CAD build for the part. Positions are in the model's coordinates, mm. A direction names the side the tool comes from. Round coordinates to 2 decimals unless told otherwise and drop trailing zeros. Order: outer loops, then holes, each group sorted by start corner. A loop starts at its lowest first (then second) coordinate and runs counter-clockwise, first axis right, second up.
Autodesk Inventor part; units mm, degrees
ref_plane "YZ Plane" through (0, 0, 0) normal (1, 0, 0) x (0, 1, 0)
ref_plane "XZ Plane" through (0, 0, 0) normal (0, 1, 0) x (-1, 0, 0)
ref_plane "XY Plane" through (0, 0, 0) normal (0, 0, 1) x (1, 0, 0)
sketch "Sketch6" plane through (0, 0, 0) normal (1, 0, 0) x (0, 1, 0)
  line L0 (0, 0) -> (12.5, 0)
  line L1 (0, 0) -> (0, -21.75)
  line L2 (0, -21.75) -> (2, -21.75)
  line L3 (2, -21.75) -> (2, -18.75)
  line L4 (2, -18.75) -> (5.5, -18.75)
  line L5 (5.5, -18.75) -> (5.5, -21.75)
  line L6 (5.5, -21.75) -> (7.5, -21.75)
  line L7 (7.5, -21.75) -> (7.5, -7)
  line L8 (7.5, -7) -> (12.5, -7)
  line L9 (12.5, -7) -> (12.5, 0)
  point P0 (6.25, 0)
  dimension "d28" = 43.5
  dimension "d29" = 14
  dimension "d30" = 5
  dimension "d31" = 7
  dimension "d33" = 3.5
  dimension "d35" = 12.5
  dimension "d36" = 37.5
revolve "Revolution3" add sketch "Sketch6" angle 360 about axis through (0, 0, 0) along (0, 1, 0)
hole "Hole2" at (0, 12.5, 0) direction (0, -1, 0) diameter 6.561 end through all
sketch "Sketch7" plane through (0, 12.5, 0) normal (0, 1, 0) x (1, 0, 0)
  circle A0 centre (0, 0) radius 7 construction
  line L0 (-4.3301, -5.5) -> (4.3301, -5.5)
  line L1 (7, 0) -> (-7, 0)
  line L2 (-4.3301, 5.5) -> (4.3301, 5.5)
  arc A1 (-4.3301, -5.5) -> (4.3301, -5.5) centre (0, 0) ccw
  arc A2 (4.3301, 5.5) -> (-4.3301, 5.5) centre (0, 0) ccw
  dimension "d49" = 11
extrude "Extrusion2" cut sketch "Sketch7" against normal up to surface (5 mm away)
chamfer "Chamfer5" distance 0.5 angle 45 6 edges at (0, 0, 21.75) (0, 7.5, 21.75) (7, 12.5, 0) (-7, 12.5, 0) (0, 0, -3.2805) (0, 12.5, -3.2805)
properties part number "Endcap" material "Steel"
1. Pin check, flat tips, straight feed: P1, Ø4, axis at x = 1.5, y = 11, coming from the -Z side; P2, Ø2, axis at y = 9, z = -4.5, coming from the -X side; P3, Ø1.5, axis at y = 3, z = 15.5, coming from the -X side; P4, Ø4, axis at x = -5.5, z = -2.5, coming from the -Y side. Stop position of each tip, or through.
2. Drill centre lines: line 1 (Z direction, x = 0, y = 6); line 2 (X direction, y = 4.25, z = 0); line 3 (X direction, y = 9.75, z = 0). Where is each one in solid material? Low to high.
3. Cut at A-A, the plane x = 0. Write the cut outline in (y, z), and give its area (3 significant figures).
4. Tool access for faces 1 (the face through (0, 10, -5.5)), 2 (the face through (7, 10, 0)), 3 (the face through (-7, 10, 0)): list every direction of +Z, -Z, +X, -X, +Y, -Y with a clear straight run to the whole face (end or side of a thin tool).
5. Cut at C-C, the plane y = 10. Write the cut outline in (x, z).
6. Mould opens along Z. For faces 4 (the face through (3.202, 6.17, -0.711)), 5 (the face through (-2, 12.5, -4)), 6 (the face through (6.64, 12.36, -0.09)) say: released by +Z, released by -Z, zero draft, split by the parting line, or undercut.
Outcome:
1. P1: stops at z = -5.5
1. P2: stops at x = -6.06
1. P3: stops at x = -11.58
1. P4: stops at y = 0
2. line 1: z = -21.75 to -3.28, 3.28 to 21.75
2. line 2: x = -18.75 to -3.28, 3.28 to 18.75
2. line 3: x = -7 to -3.28, 3.28 to 7
3. outline: (0, -21.25) - (0.5, -21.75) - (2, -21.75) - (2, -18.75) - (5.5, -18.75) - (5.5, -21.75) - (7, -21.75) - (7.5, -21.25) - (7.5, -5.5) - (12.5, -5.5) - (12.5, -3.78) - (12, -3.28) - (0.5, -3.28) - (0, -3.78) - close; (0, 3.78) - (0.5, 3.28) - (12, 3.28) - (12.5, 3.78) - (12.5, 5.5) - (7.5, 5.5) - (7.5, 21.25) - (7, 21.75) - (5.5, 21.75) - (5.5, 18.75) - (2, 18.75) - (2, 21.75) - (0.5, 21.75) - (0, 21.25) - close
3. area: 277 mm2
4. face 1: -Z, +X, -X, +Y
4. face 2: +X, +Y
4. face 3: -X, +Y
5. outline: (-4.33, -5.5) - (4.33, -5.5) arc R7 ccw to (4.33, 5.5) - (-4.33, 5.5) arc R7 ccw to start; hole circle Ø6.56 at (0, 0)
6. face 4: undercut
6. face 5: zero draft
6. face 6: split by the parting line
